```python
from build123d import *

# Parameters (mm, degrees)
BOSS_EXTRUDE1_DEPTH = 2.54
FILLET1_R           = 2.54


with BuildPart() as part:
    # Sketch2 → Boss-Extrude1 (new body)
    with BuildSketch(Plane(origin=(0, 0, 0), x_dir=(0, 0, -1), z_dir=(1, 0, 0))):
        Polygon((-45.72, 22.225), (-45.72, 7.62), (-43.18, 7.62), (-43.18, 1.4478), (-38.1, 1.4478), (-38.1, 3.175), (-35.66795, 3.175), (-35.66795, 1.4478), (-32.766, 1.4478), (-32.766, -1.4478), (-35.66795, -1.4478), (-35.66795, -3.175), (-38.1, -3.175), (-38.1, -1.4478), (-43.18, -1.4478), (-43.18, -7.62), (-45.72, -7.62), (-45.72, -22.225), (-7.62, -22.225), (-7.62, -24.765), (7.62, -24.765), (7.62, -22.225), (45.72, -22.225), (45.72, -7.62), (43.18, -7.62), (43.18, -1.4478), (38.1, -1.4478), (38.1, -3.175), (35.66795, -3.175), (35.66795, -1.4478), (32.766, -1.4478), (32.766, 1.4478), (35.66795, 1.4478), (35.66795, 3.175), (38.1, 3.175), (38.1, 1.4478), (43.18, 1.4478), (43.18, 7.62), (45.72, 7.62), (45.72, 22.225), (7.62, 22.225), (7.62, 24.765), (-7.62, 24.765), (-7.62, 22.225), align=None)
    extrude(amount=BOSS_EXTRUDE1_DEPTH)

    # Fillet1
    fillet1_edges = [part.edges().sort_by_distance(p)[0] for p in [
        (1.27, -22.225, -45.72),
        (1.27, -22.225, 45.72),
        (1.27, 22.225, 45.72),
        (1.27, 22.225, -45.72),
    ]]
    fillet(fillet1_edges, radius=FILLET1_R)


solid = part.part
```
Build history of the part. All positions in model axes, mm. A direction names the side the tool comes from. Give positions to 0.01 mm unless a question says otherwise; leave off trailing zeros. Loops run counter-clockwise (first coordinate to the right, second up) from the corner with the lowest first, then second, coordinate; pieces in that order, holes last. Notation, with made-up numbers: (32.25, 78) - (78.25, 78) arc R9 ccw to (78.25, 86) - close; hole circle Ø5 at (17.25, -29.75). An arc over 180 degrees is marked (long way). Use a Markdown table: item, result.
(1) Band-saw the part on B-B (y = -5.5). Give the cut face in (x, z), and give its area (3 significant figures).
Taken from the geometry:
| item | result |
|---|---|
| outline | (0, -43.18) - (2.54, -43.18) - (2.54, 43.18) - (0, 43.18) - close |
| area | 219 mm2 |
(2) Pull direction Z, two halves, no side cores. Call faces 6 (the face through (1, 0, -32.766)), 7 (the face through (1, -23, 7.62)), 8 (the face through (0, 0, 1)), 9 (the face through (1, -3.175, -37)): +Z half, -Z half, draft (parallel to the pull), parting line (faces both ways), or undercut.
Taken from the geometry:
| item | result |
|---|---|
| face 6 | -Z half |
| face 7 | +Z half |
| face 8 | draft |
| face 9 | undercut |
(3) Band-saw the part on A-A (z = 40.5). Give the cut face in (x, y) (3 decimals).
Taken from the geometry:
| item | result |
|---|---|
| outline | (0, -22.225) - (2.54, -22.225) - (2.54, -1.448) - (0, -1.448) - close; (0, 1.448) - (2.54, 1.448) - (2.54, 22.225) - (0, 22.225) - close |
(4) Band-saw the part on C-C (z = 21.5). Give the cut face in (x, y) (3 decimals), and give its area (3 significant figures).
Taken from the geometry:
| item | result |
|---|---|
| outline | (0, -22.225) - (2.54, -22.225) - (2.54, 22.225) - (0, 22.225) - close |
| area | 113 mm2 |
(5) Wall check: line 1 along Z through (x, y) = (1.2, 3); line 2 along Y through (x, z) = (1.65, -34) (3 decimals); line 3 along Y through (x, z) = (0.85, 32.5) (3 decimals). Give the ranges that are in metal, low to high.
Taken from the geometry:
| item | result |
|---|---|
| line 1 | -43.18 to -38.1, -35.67 to 35.67, 38.1 to 43.18 |
| line 2 | -22.225 to -1.448, 1.448 to 22.225 |
| line 3 | -22.225 to 22.225 |
(6) Drop flat-ended pins along their axis: pin 1 Ø0.9 at (x, y) = (1.5, -2.5) entering from +Z; pin 2 Ø1.2 at (x, z) = (1, -37) entering from -Y (3 decimals); pin 3 Ø0.5 at (x, y) = (1.5, -2) entering from -Z. Give the stop position or say it passes through.
Taken from the geometry:
| item | result |
|---|---|
| pin 1 | z = 43.18 |
| pin 2 | y = -22.225 |
| pin 3 | z = -43.18 |
(7) Which spindle directions (+Z, -Z, +X, -X, +Y, -Y) get a long thin tool onto all of the face, cutting with end or side? Do faces 1 (the face through (1, -2, 35.668)), 2 (the face through (1, 5, 43.18)), 3 (the face through (1, -5, -43.18)), 4 (the face through (1, 22.225, 25)), 5 (the face through (1, -24.765, 0)). Say none if no direction does.
Taken from the geometry:
| item | result |
|---|---|
| face 1 | +X, -X |
| face 2 | +Z, +X, -X |
| face 3 | -Z, +X, -X |
| face 4 | +Z, +X, -X, +Y |
| face 5 | +Z, -Z, +X, -X, -Y |
